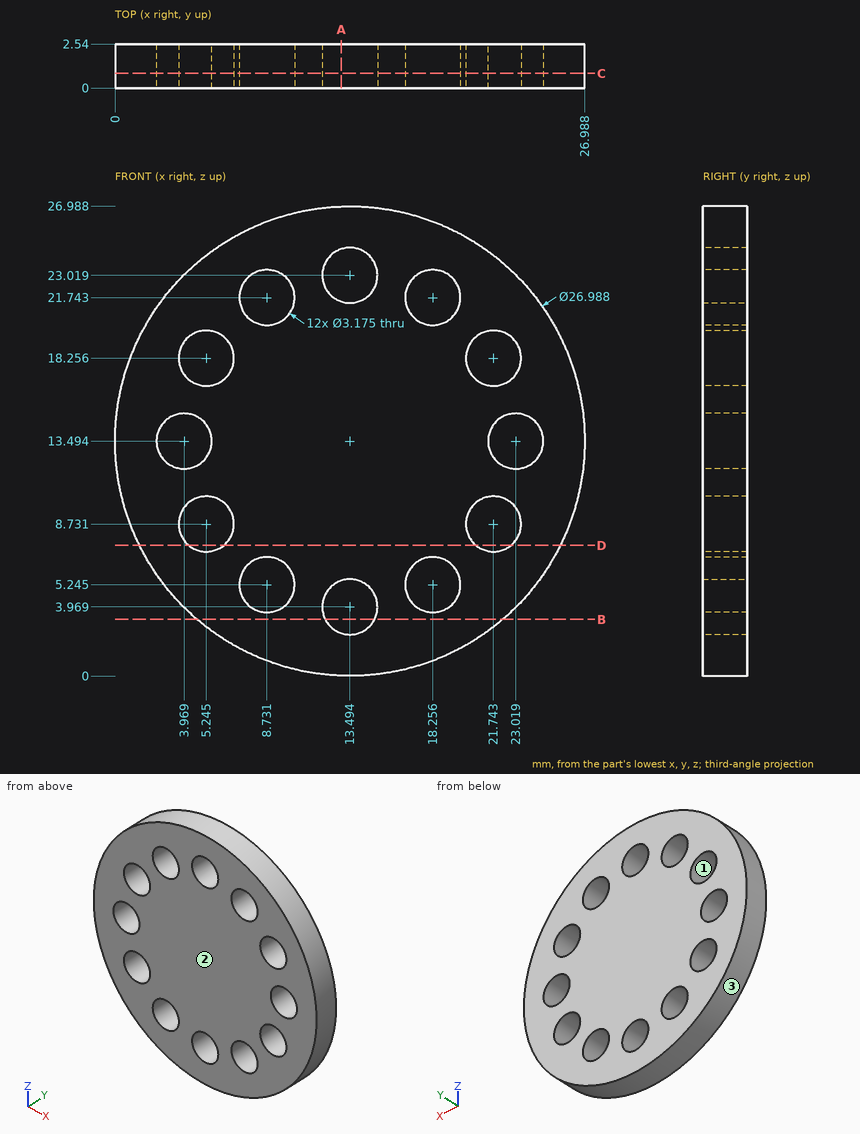
Can you work these out from the drawing? Everything is in mm from the part's minimum corner. Round coordinates to 2 decimals unless told otherwise and drop trailing zeros. Write each loop counter-clockwise with the first axis right and the second up, starting at its lowest first coordinate (ties: lowest second). Pieces come first, ordered by that corner, then holes. Notation, with made-up numbers: (36, -5.75) - (66, -5.75) arc R29 cw to (66, 29.25) - close; hole circle Ø3 at (51, 25.25). An arc over 180 degrees is marked (long way). Use a Markdown table: item, result.
Q1. I want a section at D-D (z = 7.5). List the corners of the cut face in (x, y) for me (1 decimal).
Output values:
| item | result |
|---|---|
| outline | (1.4, 0) - (4.2, 0) - (4.2, 2.5) - (1.4, 2.5) - close; (6.2, 0) - (20.7, 0) - (20.7, 2.5) - (6.2, 2.5) - close; (22.7, 0) - (25.6, 0) - (25.6, 2.5) - (22.7, 2.5) - close |
Q2. For pin 1 (1.9 mm diameter, centred on x = 5.24, z = 18.26, fed in from +Y); pin 2 (1 mm diameter, centred on x = 20.5, y = 2, fed in from -Z); pin 3 (1 mm diameter, centred on y = 1.5, z = 24, fed in from +X) (1 decimal); pin 4 (1 mm diameter, centred on x = 19, y = 1, fed in from -Z), each with a flat end and sliding along its axis, tell me the tip position at first contact or that it passes through.
Output values:
| item | result |
|---|---|
| pin 1 | through |
| pin 2 | z = 1.67 |
| pin 3 | x = 22.5 |
| pin 4 | z = 0.96 |
Q3. I want a section at C-C (y = 0.85). Count the separate pieces of the cut face and the enclosed holes in it, plus the area to 3 significant figures.
Output values:
| item | result |
|---|---|
| separate pieces | 1 |
| enclosed holes | 12 |
| area | 477 mm2 |
Q4. Please list where these lines run through material, in increasing order: L1, parallel to X at y = 1.9, z = 13.75 (1 decimal); L2, parallel to X at y = 0.1, z = 17.25 (1 decimal); L3, parallel to Z at x = 22.75, y = 0.15 (1 decimal).
Output values:
| item | result |
|---|---|
| L1 | 0 to 2.4, 5.5 to 21.5, 24.6 to 27 |
| L2 | 0.5 to 4, 6.5 to 20.5, 23 to 26.5 |
| L3 | 3.7 to 7.5, 10 to 11.9, 15.1 to 17, 19.5 to 23.3 |
Q5. Thinking about a two-plate mould opening in X: for the marked faces 1, 2 and 3, which applies, released by +X, released by -X, zero draft, split by the parting line, or undercut?
Output values:
| item | result |
|---|---|
| face 1 | undercut |
| face 2 | zero draft |
| face 3 | split by the parting line |
Q6. I want a section at A-A (x = 13). List the corners of the cut face in (y, z) for me.
Output values:
| item | result |
|---|---|
| outline | (0, 0.01) - (2.54, 0.01) - (2.54, 2.46) - (0, 2.46) - close; (0, 5.48) - (2.54, 5.48) - (2.54, 21.51) - (0, 21.51) - close; (0, 24.53) - (2.54, 24.53) - (2.54, 26.98) - (0, 26.98) - close |
Q7. I want a section at B-B (z = 3.25). List the corners of the cut face in (x, y) for me.
Output values:
| item | result |
|---|---|
| outline | (4.71, 0) - (12.08, 0) - (12.08, 2.54) - (4.71, 2.54) - close; (14.91, 0) - (22.28, 0) - (22.28, 2.54) - (14.91, 2.54) - close |
